Autodesk Inventor part; units mm, degrees
ref_plane "YZ Plane" through (0, 0, 0) normal (1, 0, 0) x (0, 1, 0)
ref_plane "XZ Plane" through (0, 0, 0) normal (0, 1, 0) x (-1, 0, 0)
ref_plane "XY Plane" through (0, 0, 0) normal (0, 0, 1) x (1, 0, 0)
sketch "Sketch1" plane through (0, 0, 0) normal (0, 1, 0) x (-1, 0, 0)
  line L0 (21.15, 45) -> (-21.15, 45)
  line L1 (-21.15, 45) -> (-21.15, -45)
  line L2 (-21.15, -45) -> (21.15, -45)
  line L3 (21.15, -45) -> (21.15, 45)
  line L4 (21.15, 45) -> (-21.15, -45) construction
  line L5 (-21.15, 45) -> (21.15, -45) construction
  point P0 (0, 0)
  dimension "d0" = 42.3
  dimension "d1" = 90
extrude "Extrusion1" add sketch "Sketch1" along normal blind 5
sketch "Sketch2" plane through (0, 5, 0) normal (0, 1, 0) x (1, 0, 0)
  line L0 (0, 0) -> (0, 42.5)
  line L1 (21.15, -45) -> (21.15, 45)
  line L2 (-21.15, 40) -> (21.15, 40)
  line L3 (21.15, 40) -> (21.15, 45)
  line L4 (21.15, 45) -> (-21.15, 45)
  line L5 (-21.15, 45) -> (-21.15, 40)
  line L6 (-21.15, 40) -> (21.15, 45) construction
  line L7 (21.15, 40) -> (-21.15, 45) construction
  dimension "d4" = 42.5
  dimension "d5" = 42.3
  dimension "d6" = 5
extrude "Extrusion2" add sketch "Sketch2" along normal blind 42.3
sketch "Sketch3" plane through (-21.15, 5, -40) normal (0, 0, 1) x (1, 0, 0)
  line L0 (42.3, 0) -> (0, 0)
  line L1 (42.3, 0) -> (42.3, 42.3)
  line L2 (0, 42.3) -> (42.3, 42.3)
  line L3 (0, 0) -> (0, 42.3)
  line L4 (42.3, 42.3) -> (0, 0)
  line L5 (5.65, 36.65) -> (36.65, 36.65)
  line L6 (36.65, 36.65) -> (36.65, 5.65)
  line L7 (36.65, 5.65) -> (5.65, 5.65)
  line L8 (5.65, 5.65) -> (5.65, 36.65)
  line L9 (5.65, 36.65) -> (36.65, 5.65) construction
  line L10 (36.65, 36.65) -> (5.65, 5.65) construction
  circle A0 centre (5.65, 36.65) radius 1.75
  circle A1 centre (36.65, 36.65) radius 1.75
  circle A2 centre (5.65, 5.65) radius 1.75
  circle A3 centre (36.65, 5.65) radius 1.75
  point P0 (21.15, -5)
  point P1 (21.15, 21.15)
  dimension "d9" = 31
  dimension "d10" = 31
  dimension "d11" = 3.5
  dimension "d14" = 31
  dimension "d17" = 31
extrude "Extrusion3" cut sketch "Sketch3" against normal blind 42.3 contours A2 L8 L4 | L4 L7 A2 | A1 L6 L4 | L4 L5 A1 | L8 A2 L4 | L4 A2 L7 | L6 A1 L4 | L4 A1 L5 | A0 L5 L8 | L8 L5 A0 | A3 L6 L7 | L7 L6 A3
chamfer "Chamfer1" distance 2 angle 45 1 edges at (0, 5, -40)
chamfer "Chamfer2" distance 2 angle 45 3 edges at (21.15, 47.3, -42.5) (-21.15, 47.3, -42.5) (0, 0, -45)
sketch "Sketch4" plane through (0, 5, 0) normal (0, 1, 0) x (1, 0, 0)
  line L0 (-21.15, -45) -> (21.15, -45)
  line L1 (0, -45) -> (0, -33)
  line L2 (0, -33) -> (0, -13)
  circle A0 centre (0, -33) radius 2
  circle A1 centre (0, -13) radius 2
  point P0 (0, 0)
  dimension "d28" = 12
  dimension "d29" = 20
  dimension "d30" = 4
  dimension "d31" = 4
sketch "Sketch5" plane through (21.15, 2, -45) normal (0, 0, -1) x (-1, 0, 0)
  circle A0 centre (5.65, 39.65) radius 1.75
  circle A1 centre (36.65, 39.65) radius 1.75
  circle A2 centre (5.65, 8.65) radius 1.75
  circle A3 centre (36.65, 8.65) radius 1.75
  circle A4 centre (5.65, 39.65) radius 2.5
  circle A5 centre (36.65, 39.65) radius 2.5
  circle A6 centre (5.65, 8.65) radius 2.5
  circle A7 centre (36.65, 8.65) radius 2.5
  point P0 (21.15, -2)
  dimension "d32" = 5
  dimension "d33" = 5
  dimension "d34" = 5
  dimension "d35" = 5
extrude "Extrusion4" cut sketch "Sketch5" against normal blind 2 contours A0 | A1 | A2 | A3 | A4 | A5 | A6 | A7
extrude "Extrusion5" cut sketch "Sketch4" against normal blind 5
fillet "Fillet1" radius 5 2 edges at (21.15, 2.5, 45) (-21.15, 2.5, 45)
properties part number "ACOPLE PARA NEMA DE CAJA"
Here's how the part is built. I have some questions about the finished solid (model axes, mm). A direction names the side the tool comes from. Round coordinates to 2 decimals unless told otherwise and drop trailing zeros. Loops run counter-clockwise (first coordinate to the right, second up) from the corner with the lowest first, then second, coordinate; pieces in that order, holes last. Notation, with made-up numbers: (34.25, 83.5) -> (65.25, 83.5) arc R10 cw to (65.25, 99.5) -> close; hole circle Ø1 at (27.25, 30.25). An arc over 180 degrees is marked (long way). Answer as CSV lines item,"result". Start each with the question number.
1. If we mould it in two halves opening along Y, with no side actions, what happens to faces 4 (the face through (20.16, 46.29, -42.46)), 5 (the face through (21.15, 4, -18)), 6 (the face through (-13.883, 9.98, -41.479)), 7 (the face through (0, 0, 2))? For each: pulls with the +Y half, pulls with the -Y half, needs draft (parallel to the pull), parting line crosses it, or undercut.
2. For faces 1 (the face through (0, 5, 4)), 2 (the face through (0, 3, 35)), 3 (the face through (14, 9, -43)), which set-ups out of +Z, -Z, +X, -X, +Y, -Y let a thin tool reach every point of the face, with its end or its side?
3. Imagine slicing it at C-C on y = 41.65. Write out the boundary of the cut face in (x, z).
4. Imagine slicing it at D-D on y = 33. Write out the boundary of the cut face in (x, z), plus the area to 4 significant figures.
5. Imagine slicing it at A-A on z = 33. Write out the boundary of the cut face in (x, y).
6. I'm going to push flat-ended pins straight in: P1, Ø5.5, axis at x = -15.5, y = 41.65, coming from the +Z side; P2, Ø1.5, axis at x = -15, y = 10.5, coming from the -Z side; P3, Ø1.5, axis at x = 11, z = 32.5, coming from the +Y side; P4, Ø1.5, axis at x = -14.5, y = 40.5, coming from the -Z side. Where does each tip first touch, or does it pass through?
7. I need wall thicknesses on probe 1 along X at (y, z) = (41.65, -42.25); probe 2 along Z at (x, y) = (0, 3.55); probe 3 along Y at (x, z) = (15.5, -41.85). Which ranges of each line are inside material? Lowest first, please. Write a range as from..to.
8. Imagine slicing it at B-B on x = 0. Write out the boundary of the cut face in (y, z), plus the area to 4 significant figures.
Solution:
1,face 4,"pulls with the +Y half"
1,face 5,"needs draft"
1,face 6,"undercut"
1,face 7,"pulls with the -Y half"
2,face 1,"+Z, +X, -X, +Y"
2,face 2,"+Y, -Y"
2,face 3,"-Z"
3,outline,"(-21.15, -45) -> (-18, -45) -> (-18, -43) -> (-17.25, -43) -> (-17.25, -40) -> (-21.15, -40) -> close; (-13.75, -43) -> (-13, -43) -> (-13, -45) -> (13, -45) -> (13, -43) -> (13.75, -43) -> (13.75, -40) -> (-13.75, -40) -> close; (17.25, -43) -> (18, -43) -> (18, -45) -> (21.15, -45) -> (21.15, -40) -> (17.25, -40) -> close"
4,outline,"(-21.15, -45) -> (21.15, -45) -> (21.15, -40) -> (-21.15, -40) -> close"
4,area,"211.5 mm²"
5,outline,"(-21.15, 0) -> (-2, 0) -> (-2, 5) -> (-21.15, 5) -> close; (2, 0) -> (21.15, 0) -> (21.15, 5) -> (2, 5) -> close"
6,P1,"z = -40"
6,P2,"through"
6,P3,"y = 5"
6,P4,"z = -43"
7,probe 1,"-21.15..-17.25, -13.75..13.75, 17.25..21.15"
7,probe 2,"-45..11, 15..31, 35..45"
7,probe 3,"0..8.9, 12.4..39.9, 43.4..47.3"
8,outline,"(0, -43) -> (2, -45) -> (47.3, -45) -> (47.3, -40) -> (7, -40) -> (5, -38) -> (5, 11) -> (0, 11) -> close; (0, 15) -> (5, 15) -> (5, 31) -> (0, 31) -> close; (0, 35) -> (5, 35) -> (5, 45) -> (0, 45) -> close"
8,area,"621.5 mm²"
